Can you work these out from the model? Positions are in its coordinate system, mm. A direction names the side the tool comes from. Give positions to 0.01 mm unless a question says otherwise; leave off trailing zeros. Write each loop counter-clockwise with the first axis right and the second up, starting at its lowest first coordinate (ties: lowest second). Pieces come first, ordered by that corner, then holes.
from build123d import *

# Parameters (mm, degrees)
BOSS_EXTRUDE1_DEPTH = 50
SKETCH2_R           = 10
BOSS_EXTRUDE2_DEPTH = 50
SKETCH3_R           = 10
BOSS_EXTRUDE3_DEPTH = 50
SKETCH4_R           = 10
BOSS_EXTRUDE4_DEPTH = 50
SKETCH5_R           = 10
BOSS_EXTRUDE5_DEPTH = 50


with BuildPart() as part:
    # Sketch1 → Boss-Extrude1 (new body)
    with BuildSketch(Plane(origin=(0, 0, 0), x_dir=(1, 0, 0), z_dir=(0, 1, 0))):
        Polygon((1413.835542094, 637.601174935), (1413.835542094, 537.601174935), (1463.835542094, 537.601174935), (1463.835542094, 627.601174935), (1523.835542094, 627.601174935), (1523.835542094, 507.601174935), (1413.835542094, 507.601174935), (1413.835542094, -367.509476585), (1463.835542094, -367.509476585), (1463.835542094, -292.398825065), (1523.835542094, -292.398825065), (1523.835542094, -412.398825065), (1413.835542094, -412.398825065), (913.835542094, -412.398825065), (803.835542094, -412.398825065), (803.835542094, -292.398825065), (863.835542094, -292.398825065), (863.835542094, -367.509476585), (913.835542094, -367.509476585), (913.835542094, 507.601174935), (803.835542094, 507.601174935), (803.835542094, 627.601174935), (863.835542094, 627.601174935), (863.835542094, 537.601174935), (913.835542094, 537.601174935), (913.835542094, 637.601174935), align=None)
    extrude(amount=BOSS_EXTRUDE1_DEPTH)

    # Sketch2 → Boss-Extrude2 (add)
    with BuildSketch(Plane(origin=(0, 0, -627.601174935), x_dir=(-1, 0, 0), z_dir=(0, 0, -1))):
        with Locations(Location((-828.835542094, 25, 0), (0, 0, 180))):
            Circle(SKETCH2_R)
    extrude(amount=BOSS_EXTRUDE2_DEPTH)

    # Sketch3 → Boss-Extrude3 (add)
    with BuildSketch(Plane(origin=(0, 0, 292.398825065), x_dir=(-1, 0, 0), z_dir=(0, 0, -1))):
        with Locations(Location((-828.835542094, 25, 0), (0, 0, 180))):
            Circle(SKETCH3_R)
    extrude(amount=BOSS_EXTRUDE3_DEPTH)

    # Sketch4 → Boss-Extrude4 (add)
    with BuildSketch(Plane(origin=(0, 0, -627.601174935), x_dir=(-1, 0, 0), z_dir=(0, 0, -1))):
        with Locations(Location((-1498.835542094, 25, 0), (0, 0, 180))):
            Circle(SKETCH4_R)
    extrude(amount=BOSS_EXTRUDE4_DEPTH)

    # Sketch5 → Boss-Extrude5 (add)
    with BuildSketch(Plane(origin=(0, 0, 292.398825065), x_dir=(-1, 0, 0), z_dir=(0, 0, -1))):
        with Locations(Location((-1498.835542094, 25, 0), (0, 0, 180))):
            Circle(SKETCH5_R)
    extrude(amount=BOSS_EXTRUDE5_DEPTH)


solid = part.part
(1) If we mould it in two halves opening along X, with no side actions, what happens to faces 1 (the face through (1499, 25, 242.399)), 2 (the face through (1160, 25, -637.601)), 3 (the face through (1523.836, 25, -568))? For each: +X half, -X half, draft (parallel to the pull), parting line (faces both ways), or undercut.
Returned:
face 1: draft
face 2: undercut
face 3: +X half
(2) Will these pins go through, and if not, where does the flat tip stop? P1, Ø15, axis at x = 1443, y = 16, coming from the -Z side; P2, Ø15, axis at y = 24, z = -161.5, coming from the +X side; P3, Ø6, axis at y = 34.5, z = 215, coming from the -X side.
Returned:
P1: stops at z = -537.6
P2: stops at x = 1413.84
P3: stops at x = 913.84
(3) For faces 4 (the face through (1508, 29, -652)), 5 (the face through (1413.836, 25, -588)), 6 (the face through (829, 25, 242.399)), 7 (the face through (1508, 29, 268)), which set-ups out of +Z, -Z, +X, -X, +Y, -Y let a thin tool reach every point of the face, with its end or its side?
Returned:
face 4: -Z
face 5: -Z, +Y, -Y
face 6: -X, +Y, -Y
face 7: none
(4) Imagine slicing it at C-C, the plane x = 1218.5. Write out the boundary of the cut face in (y, z), plus the area to 3 significant figures.
Returned:
outline: (0, -637.6) - (50, -637.6) - (50, 412.4) - (0, 412.4) - close
area: 52,500 mm2
(5) If I drill on L1, parallel to X at y = 14.5, z = 333; L2, parallel to Z at x = 1455, y = 43; L3, parallel to X at y = 5.5, z = -230.5, over which ranges is the centre line in solid material (lowest first)?
Returned:
L1: x = 803.84 to 863.84, 913.84 to 1413.84, 1463.84 to 1523.84
L2: z = -537.6 to -507.6, 367.51 to 412.4
L3: x = 913.84 to 1413.84
(6) Imagine slicing it at A-A, the plane x = 1477. Write out the boundary of the cut face in (y, z), plus the area to 3 significant figures.
Returned:
outline: (0, -627.6) - (50, -627.6) - (50, -507.6) - (0, -507.6) - close; (0, 292.4) - (50, 292.4) - (50, 412.4) - (0, 412.4) - close
area: 12,000 mm2
(7) Imagine slicing it at B-B, the plane z = 52. Write out the boundary of the cut face in (x, y).
Returned:
outline: (913.84, 0) - (1413.84, 0) - (1413.84, 50) - (913.84, 50) - close
